```python
from build123d import *

# Parameters (mm, degrees)
F0_W          = 72.2392462194
F0_H          = 16.11712249
F1_DEPTH      = 25.4
F2_W          = 15.2537054382
F2_H          = 14.6780936047
F3_DEPTH      = 50.8
F3_DEPTH_BACK = 25.4
F5_R          = 6.3741022215
F6_DEPTH      = 25.401


with BuildPart() as f1:
    # F0 (on Front) → F1 (new body)
    with BuildSketch(Plane.XZ):
        with Locations((2.8780568391, -0.4317087587)):
            Rectangle(F0_W, F0_H)
    extrude(amount=F1_DEPTH)

    # F2 (on Top) → F3 (cut, two sides)
    with BuildSketch(Plane.XY) as f3_sk:
        with Locations((-3.4536684398, -13.5268704034)):
            Rectangle(F2_W, F2_H)
    extrude(amount=-F3_DEPTH, mode=Mode.SUBTRACT)
    extrude(f3_sk.sketch, amount=F3_DEPTH_BACK, mode=Mode.SUBTRACT)

    # F5 (on face) → F6 (cut, through all)
    with BuildSketch(Plane.XZ.offset(25.4)):
        Circle(F5_R)
    extrude(amount=-F6_DEPTH, mode=Mode.SUBTRACT)


solid = f1.part
```
Geometry: final body of the model. Coordinates: model frame, mm. A direction names the side the tool comes from. Coordinates: 2 decimals unless noted, no trailing zeros. Order: outer loops, then holes, each group sorted by start corner. A loop starts at its lowest first (then second) coordinate and runs counter-clockwise, first axis right, second up. Notation, with made-up numbers: (81.25, 60) -> (99.25, 60) arc R22 ccw to (99.25, 80) -> close; hole circle Ø4 at (-6.75, 0). An arc over 180 degrees is marked (long way). Write item = value, one per line.
(1) Access query for faces 4 (the flat face through (4.173, -14, -7)), 5 (the flat face through (2, -25.4, -7)). Directions: +Z, -Z, +X, -X, +Y, -Y. A direction counts if a zero-diameter tool reaches every point of the face in a straight line with its end or side. Return the directions, or none.
Solved:
face_4 = +Z, -Z
face_5 = +Z, -Z, +X, -X, -Y
(2) Line query: line 1 (X direction, y = -18.75, z = 0); line 2 (X direction, y = -18.25, z = 6.25); line 3 (Y direction, x = -7, z = -6.25). Output: solid intervals per line, ascending.
Solved:
line_1 = -33.24 to -11.08, 6.37 to 39
line_2 = -33.24 to -11.08, 4.17 to 39
line_3 = -25.4 to -20.87, -6.19 to 0
(3) Pin query (flat end, axial travel): pin 1 Ø4 at (x, y) = (-3, -7.5) entering from -Z. Return the tip coordinate at first contact, or that it passes through.
Solved:
pin_1 = -8.49
(4) Pull-direction query (X, two-part tool) for faces 1 (the flat face through (10, -13, 7.627)), 2 (the flat face through (-33.242, -13, -1)), 3 (the cylindrical face through (5.89, -12.88, -2.44)); classes: pulls with the +X half, pulls with the -X half, needs draft (parallel to the pull), parting line crosses it, or undercut.
Solved:
face_1 = needs draft
face_2 = pulls with the -X half
face_3 = undercut
(5) Cut plane A-A on x = 0. Return loops of the section in (y, z).
Solved:
outline = (-25.4, -8.49) -> (-20.87, -8.49) -> (-20.87, -6.37) -> (-25.4, -6.37) -> close; (-25.4, 6.37) -> (-20.87, 6.37) -> (-20.87, 7.63) -> (-25.4, 7.63) -> close; (-6.19, -8.49) -> (0, -8.49) -> (0, -6.37) -> (-6.19, -6.37) -> close; (-6.19, 6.37) -> (0, 6.37) -> (0, 7.63) -> (-6.19, 7.63) -> close
(6) Cut plane B-B on z = 0. Return loops of the section in (x, y).
Solved:
outline = (-33.24, -25.4) -> (-6.37, -25.4) -> (-6.37, -20.87) -> (-11.08, -20.87) -> (-11.08, -6.19) -> (-6.37, -6.19) -> (-6.37, 0) -> (-33.24, 0) -> close; (6.37, -25.4) -> (39, -25.4) -> (39, 0) -> (6.37, 0) -> close
(7) Cut plane D-D on z = -4. Return loops of the section in (x, y).
Solved:
outline = (-33.24, -25.4) -> (-4.96, -25.4) -> (-4.96, -20.87) -> (-11.08, -20.87) -> (-11.08, -6.19) -> (-4.96, -6.19) -> (-4.96, 0) -> (-33.24, 0) -> close; (4.96, -25.4) -> (39, -25.4) -> (39, 0) -> (4.96, 0) -> close
(8) Cut plane C-C on y = -9. Return loops of the section in (x, z).
Solved:
outline = (-33.24, -8.49) -> (-11.08, -8.49) -> (-11.08, 7.63) -> (-33.24, 7.63) -> close; (4.17, -8.49) -> (39, -8.49) -> (39, 7.63) -> (4.17, 7.63) -> (4.17, 4.82) arc R6.37 cw to (4.17, -4.82) -> close
